```python
from build123d import *

# Parameters (mm, degrees)
BLANKSKE_W              = 80
BLANKSKE_H              = 7.5
BLANK_DEPTH             = 20
TOOTHCUTSIM_DEPTH       = 83.802475808
TEETHCUTS_COUNT         = 18
TEETHCUTS_PITCH         = 4.712388975
SKETCH1_W               = 20
SKETCH1_H               = 11.625
BOSS_EXTRUDE2_DEPTH     = 7.5
SKETCH3_W               = 20
SKETCH3_H               = 15
BOSS_EXTRUDE3_DEPTH     = 7.5
SKETCH4_W               = 7.5
SKETCH4_H               = 15
BOSS_EXTRUDE4_DEPTH     = 15
SKETCH8_W               = 7.5
SKETCH8_H               = 7.5
CUT_EXTRUDE1_DEPTH      = 15
CUT_EXTRUDE2_DEPTH      = 15
SKETCH10_W              = 7.5
SKETCH10_H              = 7.5
BOSS_EXTRUDE5_DEPTH     = 7.5
SKETCH11_W              = 7.5
SKETCH11_H              = 15
BOSS_EXTRUDE7_DEPTH     = 60
CUT_EXTRUDE4_DEPTH      = 116.829144109
CUT_EXTRUDE4_DEPTH_BACK = 116.829144109
SKETCH12_W              = 95
SKETCH12_H              = 10
SKETCH14_W              = 95
SKETCH14_H              = 2.5
CUT_EXTRUDE5_DEPTH      = 100
SKETCH15_W              = 67.5
SKETCH15_H              = 7.5
CUT_EXTRUDE6_DEPTH      = 122.963109177
BOSS_EXTRUDE8_START     = -7.5
BOSS_EXTRUDE8_DEPTH     = 7.5
BOSS_EXTRUDE9_DEPTH     = 1
FILLET1_R               = 2
FILLET2_R               = 2
FILLET3_R               = 2


with BuildPart() as part:
    # BlankSke → Blank (new body)
    with BuildSketch(Plane.XY):
        with Locations((40, 3.75)):
            Rectangle(BLANKSKE_W, BLANKSKE_H)
    extrude(amount=-BLANK_DEPTH)

    # TooCutSkeSim → ToothCutSim (cut, through all)
    with BuildSketch(Plane.XY):
        Polygon((0.654653055, 4.125), (-0.654653055, 4.125), (-1.892297439, 7.5254), (1.892297439, 7.5254), align=None)
    toothcutsim = extrude(amount=-TOOTHCUTSIM_DEPTH, mode=Mode.SUBTRACT)

    # TeethCuts: ToothCutSim ×18
    with Locations(*[(i * TEETHCUTS_PITCH, 0, 0) for i in range(1, TEETHCUTS_COUNT)]):
        add(toothcutsim, mode=Mode.SUBTRACT)

    # Sketch1 → Boss-Extrude2 (add)
    with BuildSketch(Plane(origin=(80, 0, 0), x_dir=(0, 0, -1), z_dir=(1, 0, 0))):
        with Locations((10, -1.6875)):
            Rectangle(SKETCH1_W, SKETCH1_H)
    extrude(amount=BOSS_EXTRUDE2_DEPTH)

    # Sketch3 → Boss-Extrude3 (add)
    with BuildSketch(Plane.ZY):
        with Locations((-10, 7.5)):
            Rectangle(SKETCH3_W, SKETCH3_H)
    extrude(amount=BOSS_EXTRUDE3_DEPTH)

    # Sketch4 → Boss-Extrude4 (add)
    with BuildSketch(Plane.XY):
        with Locations((-3.75, 7.5)):
            Rectangle(SKETCH4_W, SKETCH4_H)
    extrude(amount=BOSS_EXTRUDE4_DEPTH)

    # Sketch8 → Cut-Extrude1 (cut)
    with BuildSketch(Plane(origin=(0, 0, 0), x_dir=(0, 0, -1), z_dir=(1, 0, 0))):
        with Locations((-3.75, 3.75)):
            Rectangle(SKETCH8_W, SKETCH8_H)
    extrude(amount=-CUT_EXTRUDE1_DEPTH, mode=Mode.SUBTRACT)

    # Sketch9 → Cut-Extrude2 (cut)
    with BuildSketch(Plane.ZY.offset(7.5)):
        Polygon((7.5, 15), (15, 7.5), (15, 15), align=None)
    extrude(amount=-CUT_EXTRUDE2_DEPTH, mode=Mode.SUBTRACT)

    # Sketch10 → Boss-Extrude5 (add)
    with BuildSketch(Plane.XZ):
        with Locations((-3.75, 11.25)):
            Rectangle(SKETCH10_W, SKETCH10_H)
    extrude(amount=BOSS_EXTRUDE5_DEPTH)

    # Sketch11 → Boss-Extrude7 (add)
    with BuildSketch(Plane.XY.offset(15)):
        with Locations((-3.75, 0)):
            Rectangle(SKETCH11_W, SKETCH11_H)
    extrude(amount=BOSS_EXTRUDE7_DEPTH)

    # Sketch12 → Cut-Extrude4 (cut, two sides: drawn at the far end of the back side and taken through both)
    with BuildSketch(Plane(origin=(0, 4.125, 0), x_dir=(1, 0, 0), z_dir=(0, 1, 0)).offset(-CUT_EXTRUDE4_DEPTH_BACK)):
        with Locations((40, 15)):
            Rectangle(SKETCH12_W, SKETCH12_H)
    extrude(amount=CUT_EXTRUDE4_DEPTH + CUT_EXTRUDE4_DEPTH_BACK, mode=Mode.SUBTRACT)

    # Sketch14 → Cut-Extrude5 (cut)
    with BuildSketch(Plane(origin=(0, 15, 0), x_dir=(1, 0, 0), z_dir=(0, 1, 0))):
        with Locations((40, 8.75)):
            Rectangle(SKETCH14_W, SKETCH14_H)
    extrude(amount=-CUT_EXTRUDE5_DEPTH, mode=Mode.SUBTRACT)

    # Sketch15 → Cut-Extrude6 (cut, through all)
    with BuildSketch(Plane.ZY.offset(7.5)):
        with Locations((41.25, -3.75)):
            Rectangle(SKETCH15_W, SKETCH15_H)
    extrude(amount=-CUT_EXTRUDE6_DEPTH, mode=Mode.SUBTRACT)

    # Sketch16 → Boss-Extrude8 (add)
    with BuildSketch(Plane.ZY.offset(7.5).offset(BOSS_EXTRUDE8_START)):
        with BuildLine():
            ThreePointArc((15, 7.5), (12.803300859, 12.803300859), (7.5, 15))
            Line((7.5, 15), (15, 7.5))
        make_face()
    extrude(amount=BOSS_EXTRUDE8_DEPTH)

    # Sketch19 → Boss-Extrude9 (add)
    with BuildSketch(Plane.XY):
        Polygon((-7.5, 0), (-7.5, 7.5), (0, 7.5), (0, 4.125), (87.5, 4.125), (87.5, -7.5), (80, -7.5), (80, 0), align=None)
    extrude(amount=BOSS_EXTRUDE9_DEPTH)

    # Fillet1
    fillet1_edges = [part.edges().sort_by_distance(p)[0] for p in [
        (-7.5, 15, 0),
        (-7.5, 7.5, 45),
        (-7.5, 12.803300859, 12.803300859),
    ]]
    fillet(fillet1_edges, radius=FILLET1_R)

    # Fillet2
    fillet2_edges = [part.edges().sort_by_distance(p)[0] for p in [
        (-2.75, 7.5, 75),
        (-3.75, 0, 75),
        (-7.5, 0, 41.25),
        (-7.5, 2.75, 75),
        (-6.914213562, 6.914213562, 75),
    ]]
    fillet(fillet2_edges, radius=FILLET2_R)

    # Fillet3
    fillet3_edges = [part.edges().sort_by_distance(p)[0] for p in [
        (87.5, 4.125, -3.25),
    ]]
    fillet(fillet3_edges, radius=FILLET3_R)


solid = part.part
```
Here's how the part is built. I have some questions about the finished solid (model axes, mm). A direction names the side the tool comes from. Give positions to 0.01 mm unless a question says otherwise; leave off trailing zeros. Order: outer loops, then holes, each group sorted by start corner. A loop starts at its lowest first (then second) coordinate and runs counter-clockwise, first axis right, second up. Notation, with made-up numbers: (37.5, 21.25) - (61.5, 21.25) arc R15 ccw to (61.5, 41.25) - close; hole circle Ø3 at (1, 81). An arc over 180 degrees is marked (long way). Answer as a JSON object with one key per item and string values. Group by question number.
Item 1: Which directions (+Z, -Z, +X, -X, +Y, -Y) give clear straight access to the entire face, cutting with the end or side of a thin tool? Please do faces 1 (the flat face through (50, 5, 0)), 2 (the cylindrical face through (-2.712, 12.745, 12.861)), 3 (the flat face through (10.702, 5.836, -3.698)).
Item 2: Please list where these lines run through material, in increasing order: probe 1 along Z at (x, y) = (6.5, 5.25); probe 2 along Z at (x, y) = (82, -6.5).
Item 3: If we mould it in two halves opening along X, with no side actions, what happens to faces 4 (the flat face through (45, 5, 0)), 5 (the flat face through (57.826, 5.836, -3.698)), 6 (the flat face through (78.85, 5.79, -3.7))? For each: pulls with the +X half, pulls with the -X half, needs draft (parallel to the pull), parting line crosses it, or undercut.
Item 4: If we section it at A-A on z = 51: Please give me the cut outline in (x, y).
Item 5: For P1, Ø6, axis at x = -1.5, z = 53.5, coming from the -Y side; P2, Ø2.5, axis at x = 59, y = 6, coming from the +Z side; P3, Ø1, axis at y = 9.5, z = 52, coming from the -X side; P4, Ø0.8, axis at x = 78, z = -5, coming from the +Y side, each with a flat end and sliding along its axis, tell me the tip position at first contact or that it passes through.
Item 6: If we section it at B-B on y = -1.25: Please give me the cut outline in (x, z).
Result set:
{
 "1": {"face 1": "+Z, +X, +Y", "face 2": "+Z, +X, -X, +Y", "face 3": "+Z, -Z, +Y"},
 "2": {"probe 1": "-7.5 to 0", "probe 2": "-7.5 to 1"},
 "3": {"face 4": "needs draft", "face 5": "undercut", "face 6": "pulls with the +X half"},
 "4": {"outline": "(-7.5, 2) arc R2 ccw to (-5.5, 0) - (0, 0) - (0, 7.5) - (-5.5, 7.5) arc R2 ccw to (-7.5, 5.5) - close"},
 "5": {"P1": "y = 0", "P2": "z = 0", "P3": "through", "P4": "y = 7.5"},
 "6": {"outline": "(80, -7.5) - (87.5, -7.5) - (87.5, 1) - (80, 1) - close"}
}
